Design review of the part built by this model. Coordinates are the model's own, in mm. Coordinates: 2 decimals unless noted, no trailing zeros. Loops run counter-clockwise (first coordinate to the right, second up) from the corner with the lowest first, then second, coordinate; pieces in that order, holes last. Notation, with made-up numbers: M 18.25,65.25 L 76.25,65.25 A12 cw 76.25,74.25 Z; hole C 62,73 d8. An arc over 180 degrees is marked long. Answer as a JSON object with one key per item and string values. Group by question number.
1. Consider section A-A (z = 13.5). State the section outline as (x, y) points, then the cut area to 3 significant figures.
2. To check wall thickness, follow probe 1 along X at (y, z) = (5.5, 18.5); probe 2 along Y at (x, z) = (0.5, 41); probe 3 along X at (y, z) = (-5.25, 20.5). State the ranges of each line that lie inside material, in increasing order.
3. Consider section B-B (y = -4.5). State the section outline as (x, z) points.
4. Insertion check: pin 1 (2 mm diameter, centred on x = 3.5, z = 6, fed in from -Y); pin 2 (8 mm diameter, centred on x = -2, z = 42.5, fed in from +Y); pin 3 (8 mm diameter, centred on x = -3, z = 15, fed in from -Y). Each pin has a flat end and moves straight along its axis. Give the tip position at first contact, or say it passes through.
from build123d import *

# Parameters (mm, degrees)
F0_W     = 20
F0_H     = 20
F1_DEPTH = 50
F3_DEPTH = 25
F5_DEPTH = 12.5


with BuildPart() as f1:
    # F0 (on Top) → F1 (new body)
    with BuildSketch(Plane.XY):
        Rectangle(F0_W, F0_H)
    extrude(amount=F1_DEPTH)

    # F2 (on face) → F3 (cut)
    with BuildSketch(Plane.XZ.offset(10)):
        Polygon((-10, 50), (-10, 0), (0, 50), align=None)
        Polygon((0, 50), (10, 0), (10, 50), align=None)
    extrude(amount=-F3_DEPTH, mode=Mode.SUBTRACT)

    # F4 (on Right) → F5 (cut, symmetric)
    with BuildSketch(Plane.YZ):
        Polygon((0, 50), (10, 0), (10, 50), align=None)
        Polygon((-10, 50), (-10, 0), (0, 50), align=None)
    extrude(amount=F5_DEPTH, both=True, mode=Mode.SUBTRACT)


solid = f1.part
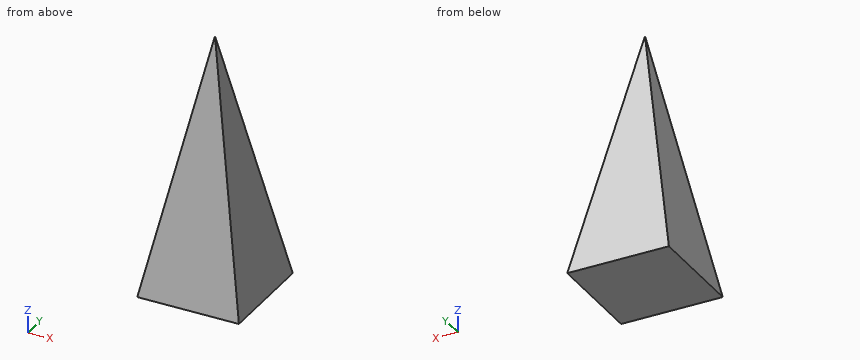
Findings below:
{
 "1": {"outline": "M -7.3,-7.3 L 7.3,-7.3 L 7.3,7.3 L -7.3,7.3 Z", "area": "213 mm^2"},
 "2": {"probe 1": "x = -6.3 to 6.3", "probe 2": "y = -1.8 to 1.8", "probe 3": "x = -5.9 to 5.9"},
 "3": {"outline": "M -10,0 L 10,0 L 4.5,27.5 L -4.5,27.5 Z"},
 "4": {"pin 1": "stops at y = -9", "pin 2": "stops at y = 2.3", "pin 3": "stops at y = -7.8"}
}
